Read the model definition and answer for the solid it produces. Units are mm, in the model's axes. A direction names the side the tool comes from. Give positions to 0.01 mm unless a question says otherwise; leave off trailing zeros. Write each loop counter-clockwise with the first axis right and the second up, starting at its lowest first coordinate (ties: lowest second). Pieces come first, ordered by that corner, then holes. Notation, with made-up numbers: (54, 54.25) - (104, 54.25) arc R4 cw to (104, 59.25) - close; hole circle Ø9 at (82, 67.5). An arc over 180 degrees is marked (long way). Use CSV: the item, a comma, the result in double quotes. Start each with the question number.
from build123d import *

# Parameters (mm, degrees)
SKETCH1_W           = 20
SKETCH1_H           = 10
BOSS_EXTRUDE1_DEPTH = 3
SKETCH2_R           = 1.5
BOSS_EXTRUDE2_DEPTH = 60
SKETCH3_R           = 1.5
BOSS_EXTRUDE3_DEPTH = 5


with BuildPart() as part:
    # Sketch1 → Boss-Extrude1 (new body)
    with BuildSketch(Plane(origin=(0, 0, 0), x_dir=(1, 0, 0), z_dir=(0, 1, 0))):
        Rectangle(SKETCH1_W, SKETCH1_H)
    extrude(amount=BOSS_EXTRUDE1_DEPTH)

    # Sketch2 → Boss-Extrude2 (add)
    with BuildSketch(Plane(origin=(0, 3, 0), x_dir=(1, 0, 0), z_dir=(0, 1, 0))):
        with Locations((-5, 0)):
            Circle(SKETCH2_R)
        with Locations((5, 0)):
            Circle(SKETCH2_R)
    extrude(amount=BOSS_EXTRUDE2_DEPTH)

    # Sketch3 → Boss-Extrude3 (add)
    with BuildSketch(Plane.XZ):
        Circle(SKETCH3_R)
    extrude(amount=BOSS_EXTRUDE3_DEPTH)


solid = part.part
(1) Which of the six approach directions +Z, -Z, +X, -X, +Y, -Y give full straight-line access (tool end or side, diameter ignored) to faces 4 (the face through (-6.2, 32.6, 0.9)), 5 (the face through (0, 1, -5))?
(2) Given P1, Ø4, axis at x = 7, z = 3.5, coming from the +Y side; P2, Ø12, axis at x = 4, y = 39, coming from the -Z side; P3, Ø6, axis at y = 51, z = 0.5, coming from the +X side, each flat-ended and moving along its own axis, determine where each tip first touches the part or whether it passes through.
(3) The part is cut by section C-C on z = -4. Write down the section's boundary in (x, y).
(4) Consider probe 1 along Y at (x, z) = (0.5, -1.25); probe 2 along Y at (x, z) = (-6.25, -0.75); probe 3 along X at (y, z) = (49.5, -1). Determine where each line is inside the solid, lowest interval first.
(5) The part is cut by section B-B on x = 5. Write down the section's boundary in (y, z).
(6) The part is cut by section D-D on x = 0. Write down the section's boundary in (y, z), plus the area to 3 significant figures.
(7) For a pull along X with two mould halves and no side action, classify faces 1 (the face through (-1.5, -2.46, 0.07)), 2 (the face through (6.386, 32.58, 0.575)), 3 (the face through (-10, 1, 0)) as pulls with the +X half, pulls with the -X half, needs draft (parallel to the pull), parting line crosses it, or undercut.
(8) The part is cut by section A-A on y = 58.5. Write down the section's boundary in (x, z).
Reported:
1,face 4,"+Y"
1,face 5,"-Z, +X, -X, +Y, -Y"
2,P1,"y = 3"
2,P2,"z = -1.5"
2,P3,"x = 6.5"
3,outline,"(-10, 0) - (10, 0) - (10, 3) - (-10, 3) - close"
4,probe 1,"-5 to 3"
4,probe 2,"0 to 63"
4,probe 3,"-6.12 to -3.88, 3.88 to 6.12"
5,outline,"(0, -5) - (3, -5) - (3, -1.5) - (63, -1.5) - (63, 1.5) - (3, 1.5) - (3, 5) - (0, 5) - close"
6,outline,"(-5, -1.5) - (0, -1.5) - (0, -5) - (3, -5) - (3, 5) - (0, 5) - (0, 1.5) - (-5, 1.5) - close"
6,area,"45.0 mm²"
7,face 1,"parting line crosses it"
7,face 2,"undercut"
7,face 3,"pulls with the -X half"
8,outline,"circle Ø3 at (-5, 0); circle Ø3 at (5, 0)"
